Verification items for the finished model (mm, model axes). Coordinates: 2 decimals unless noted, no trailing zeros. Use CSV: the item, a comma, the result in double quotes. Start each with the question number.
1) Release check for a two-part mould opening along X. For faces 1 (the cylindrical face through (-341.37, -13.17, 3.22)), 2 (the flat face through (-6, 7, 6.35)) record: released by +X, released by -X, zero draft, split by the parting line, or undercut.
2) Sectioned sample at A-A on z = 4.25. Give the number of separate pieces and of enclosed holes in the cut face, then the cut area to 3 significant figures.
3) Scan lines: line 1 along Y through (x, z) = (-114.3, 3.5); line 2 along X through (y, z) = (-11.5, 1.5); line 3 along X through (y, z) = (-12, 3). Record each from-to range of solid material in increasing order.
from build123d import *

# Parameters (mm, degrees)
SKETCH1_W           = 838.2
SKETCH1_H           = 127
BOSS_EXTRUDE1_DEPTH = 6.35
SKETCH2_R           = 14.2875
CUT_EXTRUDE1_DEPTH  = 6.35
SKETCH3_R           = 14.2875
CUT_EXTRUDE2_DEPTH  = 6.35
SKETCH4_R           = 2.5527
CUT_EXTRUDE3_DEPTH  = 6.35
SKETCH5_R           = 2.5527
CUT_EXTRUDE4_DEPTH  = 6.35
FILLET3_R           = 12.7
SKETCH6_R           = 2.5527
CUT_EXTRUDE5_DEPTH  = 6.35


with BuildPart() as part:
    # Sketch1 → Boss-Extrude1 (new body)
    with BuildSketch(Plane.XY):
        with Locations((0, 6.35)):
            Rectangle(SKETCH1_W, SKETCH1_H)
    extrude(amount=BOSS_EXTRUDE1_DEPTH)

    # Sketch2 → Cut-Extrude1 (cut)
    with BuildSketch(Plane.XY.offset(6.35)):
        with Locations((0, -19.05)):
            Circle(SKETCH2_R)
    extrude(amount=-CUT_EXTRUDE1_DEPTH, mode=Mode.SUBTRACT)

    # Sketch3 → Cut-Extrude2 (cut)
    with BuildSketch(Plane.XY.offset(6.35)):
        with Locations((-354.99802, -17.4625)):
            Circle(SKETCH3_R)
        with Locations((354.99802, -17.4625)):
            Circle(SKETCH3_R)
    extrude(amount=-CUT_EXTRUDE2_DEPTH, mode=Mode.SUBTRACT)

    # Sketch4 → Cut-Extrude3 (cut)
    with BuildSketch(Plane.XY.offset(6.35)):
        with Locations((-35.41268, 49.5808)):
            Circle(SKETCH4_R)
        with Locations((-57.15, -19.05)):
            Circle(SKETCH4_R)
        with Locations((57.15, -19.05)):
            Circle(SKETCH4_R)
        with Locations((35.41268, 49.5808)):
            Circle(SKETCH4_R)
    extrude(amount=-CUT_EXTRUDE3_DEPTH, mode=Mode.SUBTRACT)

    # Sketch5 → Cut-Extrude4 (cut)
    with BuildSketch(Plane.XY.offset(6.35)):
        with Locations((-405.79802, 33.3375)):
            Circle(SKETCH5_R)
        with Locations((408.97302, -46.0375)):
            Circle(SKETCH5_R)
        with Locations((405.79802, 33.3375)):
            Circle(SKETCH5_R)
        with Locations((63.5, -44.45)):
            Circle(SKETCH5_R)
        with Locations((-63.5, -44.45)):
            Circle(SKETCH5_R)
        with Locations((-297.84802, -42.8625)):
            Circle(SKETCH5_R)
        with Locations((297.84802, -42.8625)):
            Circle(SKETCH5_R)
        with Locations((-408.97302, -46.0375)):
            Circle(SKETCH5_R)
        with Locations((-297.84802, 33.3375)):
            Circle(SKETCH5_R)
        with Locations((297.84802, 33.3375)):
            Circle(SKETCH5_R)
        with Locations((82.55, 31.75)):
            Circle(SKETCH5_R)
        with Locations((-82.55, 31.75)):
            Circle(SKETCH5_R)
    extrude(amount=-CUT_EXTRUDE4_DEPTH, mode=Mode.SUBTRACT)

    # Fillet3
    fillet3_edges = [part.edges().sort_by_distance(p)[0] for p in [
        (-419.1, 69.85, 3.175),
        (419.1, 69.85, 3.175),
        (419.1, -57.15, 3.175),
        (-419.1, -57.15, 3.175),
    ]]
    fillet(fillet3_edges, radius=FILLET3_R)

    # Sketch6 → Cut-Extrude5 (cut)
    with BuildSketch(Plane.XY.offset(6.35)):
        with Locations((-406.4, 6.35)):
            Circle(SKETCH6_R)
        with Locations((406.4, 6.35)):
            Circle(SKETCH6_R)
        with Locations((-114.3, 57.15)):
            Circle(SKETCH6_R)
        with Locations((-114.3, -19.05)):
            Circle(SKETCH6_R)
        with Locations((114.3, 57.15)):
            Circle(SKETCH6_R)
        with Locations((114.3, -19.05)):
            Circle(SKETCH6_R)
    extrude(amount=-CUT_EXTRUDE5_DEPTH, mode=Mode.SUBTRACT)


solid = part.part
Answers follow:
1,face 1,"undercut"
1,face 2,"zero draft"
2,separate pieces,"1"
2,enclosed holes,"25"
2,area,"104,000 mm²"
3,line 1,"y = -57.15 to -21.6, -16.5 to 54.6, 59.7 to 69.85"
3,line 2,"x = -419.1 to -367.98, -342.01 to -12.13, 12.13 to 342.01, 367.98 to 419.1"
3,line 3,"x = -419.1 to -368.2, -341.8 to -12.43, 12.43 to 341.8, 368.2 to 419.1"
